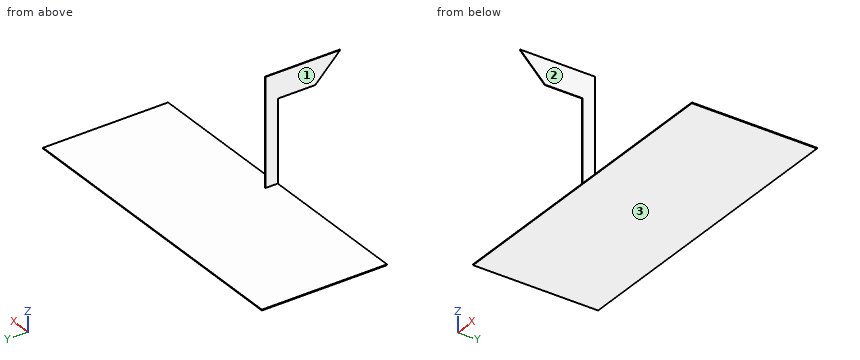
```python
from build123d import *

# Parameters (mm, degrees)
F0_W     = 1270
F0_H     = 508
F1_DEPTH = 3.175
F3_DEPTH = 1.27


with BuildPart() as f1:
    # F0 (on Top) → F1 (new body)
    with BuildSketch(Plane.XY):
        Rectangle(F0_W, F0_H)
    extrude(amount=F1_DEPTH)

    # F2 (on Right) → F3 (join, symmetric)
    with BuildSketch(Plane.YZ):
        Polygon((-254, 333.375), (-254, 3.175), (-203.2, 3.175), (-203.2, 434.975), (-508, 434.975), (-406.4, 333.375), align=None)
    extrude(amount=F3_DEPTH, both=True)


solid = f1.part
```
Verification items for the finished model (mm, model axes). Face numbers are marked on the shaded views. A direction names the side the tool comes from. Coordinates: 2 decimals unless noted, no trailing zeros. Loops run counter-clockwise (first coordinate to the right, second up) from the corner with the lowest first, then second, coordinate; pieces in that order, holes last. Notation, with made-up numbers: (-7, -26.5) -> (23, -26.5) arc R20 ccw to (23, -8.5) -> close; hole circle Ø10 at (16, 50). An arc over 180 degrees is marked (long way). Answer in a Markdown table with one row per item.
1) Depth check by flat-ended pin: P1, Ø3, axis at x = 0, y = -343.5, coming from the -Z side (3 decimals); P2, Ø2, axis at x = 0.5, z = 312.5, coming from the +Y side; P3, Ø4, axis at x = -77, y = -51, coming from the +Z side (3 decimals). Enter the tip coordinate at first touch or a pass-through.
The answers:
| item | result |
|---|---|
| P1 | stops at z = 333.375 |
| P2 | stops at y = -203.2 |
| P3 | stops at z = 3.175 |
2) Section check A-A (y = 79.5). Record the cut outline in (x, z) (3 decimals), and give its area (3 significant figures).
The answers:
| item | result |
|---|---|
| outline | (-635, 0) -> (635, 0) -> (635, 3.175) -> (-635, 3.175) -> close |
| area | 4,030 mm2 |
3) Access from +Z, -Z, +X, -X, +Y, -Y to the whole of each face (thin tool, end or side, straight path). Record for the marked faces 1, 2 and 3.
The answers:
| item | result |
|---|---|
| face 1 | +Z, -X, +Y, -Y |
| face 2 | +Z, +X, +Y, -Y |
| face 3 | -Z, +X, -X, +Y, -Y |
4) Section check B-B (z = 246.5). Record the cut outline in (x, y).
The answers:
| item | result |
|---|---|
| outline | (-1.27, -254) -> (1.27, -254) -> (1.27, -203.2) -> (-1.27, -203.2) -> close |
5) Scan lines: line 1 along Z through (x, y) = (-312, 220) (3 decimals); line 2 along X through (y, z) = (-204, 407.5). Record each from-to range of solid material in increasing order. Write a range as from..to.
The answers:
| item | result |
|---|---|
| line 1 | z = 0..3.175 |
| line 2 | x = -1.27..1.27 |
